Here's how the part is built. I have some questions about the finished solid (model axes, mm). Face numbers are marked on the shaded views. Coordinates: 2 decimals unless noted, no trailing zeros. Order: outer loops, then holes, each group sorted by start corner. A loop starts at its lowest first (then second) coordinate and runs counter-clockwise, first axis right, second up. Notation, with made-up numbers: (22.5, -19) - (52.5, -19) arc R24 cw to (52.5, -9) - close; hole circle Ø7 at (18, 11.25). An arc over 180 degrees is marked (long way). Answer as CSV lines item,"result". Start each with the question number.
Q1. Thinking about a two-plate mould opening in X: for the marked faces 1, 2, 3 and 4, which applies, released by +X, released by -X, zero draft, split by the parting line, or undercut?
Q2. Suppose I cut it at A-A (x = 0). Please give me the cut outline in (y, z).
Q3. Suppose I cut it at C-C (y = 151). Please give me the cut outline in (x, z), then the cut area to 3 significant figures.
Q4. Suppose I cut it at B-B (z = 4). Please give me the cut outline in (x, y).
Q5. I need wall thicknesses on line 1 (X direction, y = 67.5, z = -3); line 2 (Z direction, x = -12.5, y = 89); line 3 (X direction, y = 197.5, z = -0.25). Which ranges of each line are inside material? Lowest first, please.
Q6. For pin 1 Ø1.6 at (y, z) = (79, 9.5) entering from -X; pin 2 Ø3 at (x, y) = (17, 132) entering from +Z; pin 3 Ø0.6 at (y, z) = (74.5, 10.5) entering from +X; pin 4 Ø10 at (x, z) = (-3.5, -8.5) entering from -Y, each with a flat end and sliding along its axis, tell me the tip position at first contact or that it passes through.
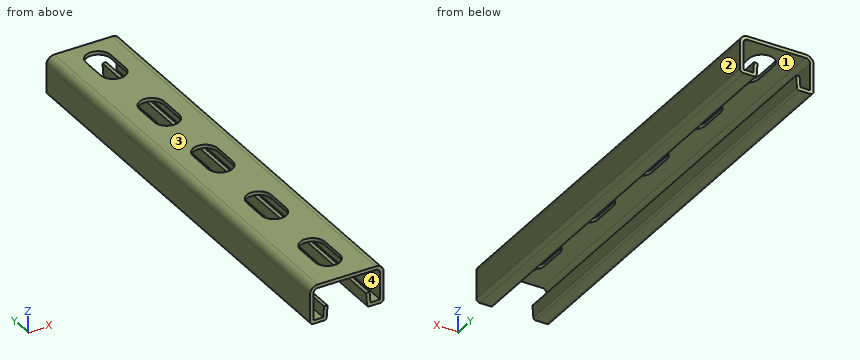
from build123d import *

# Parameters (mm, degrees)
BEAM_DEPTH          = 250
PUNCH_DEPTH         = 252.110782325
PATTERN_PUNCH_COUNT = 5
PATTERN_PUNCH_PITCH = 50.8


with BuildPart() as part:
    # sk_profile → beam (new body)
    with BuildSketch(Plane(origin=(0, 0, 0), x_dir=(1, 0, 0), z_dir=(0, 1, 0))):
        with BuildLine():
            Line((0, -10.85), (16.45, -10.85))
            ThreePointArc((16.45, -10.85), (19.631980515, -9.531980515), (20.95, -6.35))
            Line((20.95, -6.35), (20.95, 8.85))
            ThreePointArc((20.95, 8.85), (20.364213562, 10.264213562), (18.95, 10.85))
            Line((18.95, 10.85), (12.628432599, 10.85))
            ThreePointArc((12.628432599, 10.85), (11.810034567, 10.527624442), (11.431355739, 9.733707768))
            Line((11.431355739, 9.733707768), (10.95, 2.85))
            Line((10.95, 2.85), (12.945128101, 2.710487053))
            Line((12.945128101, 2.710487053), (13.374444668, 8.85))
            Line((13.374444668, 8.85), (18.95, 8.85))
            Line((18.95, 8.85), (18.95, -6.35))
            ThreePointArc((18.95, -6.35), (18.217766953, -8.117766953), (16.45, -8.85))
            Line((16.45, -8.85), (0, -8.85))
            Line((0, -8.85), (0, -10.85))
        make_face()
    beam = extrude(amount=BEAM_DEPTH)

    # mirror_half: beam across plane
    add(beam.mirror(Plane(origin=(0, 0, 0), x_dir=(0, 0, 1), z_dir=(1, 0, 0))))

    # Sketch4 → punch (cut, through all)
    with BuildSketch(Plane.XY):
        with BuildLine():
            Line((-7, 18.4), (-7, 32.4))
            ThreePointArc((-7, 32.4), (0, 39.4), (7, 32.4))
            Line((7, 32.4), (7, 18.4))
            ThreePointArc((7, 18.4), (0, 11.4), (-7, 18.4))
        make_face()
    punch = extrude(amount=PUNCH_DEPTH, mode=Mode.SUBTRACT)

    # pattern_punch: punch ×5
    with Locations(*[(0, i * PATTERN_PUNCH_PITCH, 0) for i in range(1, PATTERN_PUNCH_COUNT)]):
        add(punch, mode=Mode.SUBTRACT)


solid = part.part
Here are the results:
1,face 1,"undercut"
1,face 2,"released by +X"
1,face 3,"zero draft"
1,face 4,"undercut"
2,outline,"(0, 8.85) - (11.4, 8.85) - (11.4, 10.85) - (0, 10.85) - close; (39.4, 8.85) - (62.2, 8.85) - (62.2, 10.85) - (39.4, 10.85) - close; (90.2, 8.85) - (113, 8.85) - (113, 10.85) - (90.2, 10.85) - close; (141, 8.85) - (163.8, 8.85) - (163.8, 10.85) - (141, 10.85) - close; (191.8, 8.85) - (214.6, 8.85) - (214.6, 10.85) - (191.8, 10.85) - close; (242.6, 8.85) - (250, 8.85) - (250, 10.85) - (242.6, 10.85) - close"
3,outline,"(-20.95, -8.85) arc R2 ccw to (-18.95, -10.85) - (-12.63, -10.85) arc R1.2 ccw to (-11.43, -9.73) - (-10.95, -2.85) - (-12.95, -2.71) - (-13.37, -8.85) - (-18.95, -8.85) - (-18.95, 6.35) arc R2.5 cw to (-16.45, 8.85) - (16.45, 8.85) arc R2.5 cw to (18.95, 6.35) - (18.95, -8.85) - (13.37, -8.85) - (12.95, -2.71) - (10.95, -2.85) - (11.43, -9.73) arc R1.2 ccw to (12.63, -10.85) - (18.95, -10.85) arc R2 ccw to (20.95, -8.85) - (20.95, 6.35) arc R4.5 ccw to (16.45, 10.85) - (-16.45, 10.85) arc R4.5 ccw to (-20.95, 6.35) - close"
3,area,"209 mm²"
4,outline,"(-20.95, 0) - (-18.95, 0) - (-18.95, 250) - (-20.95, 250) - close; (18.95, 0) - (20.95, 0) - (20.95, 250) - (18.95, 250) - close"
5,line 1,"x = -20.95 to -18.95, -12.97 to -10.96, 10.96 to 12.97, 18.95 to 20.95"
5,line 2,"z = -10.84 to -2.74, 8.85 to 10.85"
5,line 3,"x = -20.95 to -18.95, 18.95 to 20.95"
6,pin 1,"stops at x = -20.29"
6,pin 2,"stops at z = 10.85"
6,pin 3,"stops at x = 18.78"
6,pin 4,"passes through"
